CAD build for the part. Positions are in the model's coordinates, mm. Face numbers are marked on the shaded views. A direction names the side the tool comes from. Coordinates: 2 decimals unless noted, no trailing zeros. Order: outer loops, then holes, each group sorted by start corner. A loop starts at its lowest first (then second) coordinate and runs counter-clockwise, first axis right, second up. Notation, with made-up numbers: M 79,11.5 L 134,11.5 A20 ccw 134,44.5 Z; hole C 49,80 d8. An arc over 180 degrees is marked long. Write item = value, one per line.
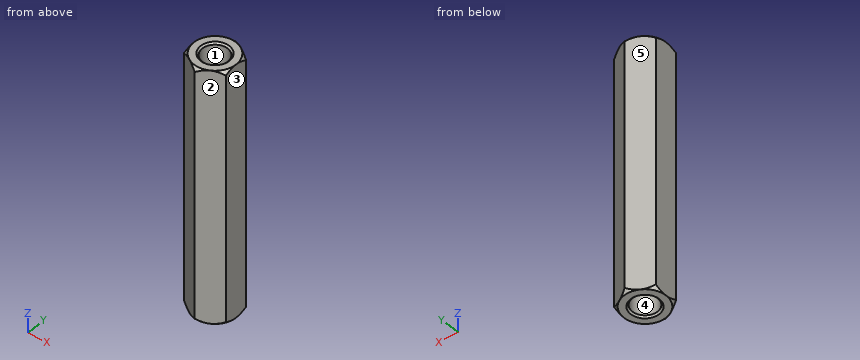
Autodesk Inventor part; units mm, degrees
ref_plane "Pracovní rovina1" through (0, 0, 15) normal (0, 0, -1) x (-1, 0, 0)
ref_plane "YZ Plane" through (0, 0, 0) normal (1, 0, 0) x (0, 1, 0)
ref_plane "XZ Plane" through (0, 0, 0) normal (0, 1, 0) x (-1, 0, 0)
sketch "Náčrt1" plane through (0, 0, 0) normal (0, 0, 1) x (1, 0, 0)
  line L0 (2.5, -1.4434) -> (0, -2.8868)
  line L1 (0, -2.8868) -> (-2.5, -1.4434)
  line L2 (-2.5, -1.4434) -> (-2.5, 1.4434)
  line L3 (-2.5, 1.4434) -> (0, 2.8868)
  line L4 (0, 2.8868) -> (2.5, 1.4434)
  line L5 (2.5, 1.4434) -> (2.5, -1.4434)
  circle A0 centre (0, 0) radius 1.5
  point P0 (2.5, 0)
  dimension "d1" = 3
  dimension "d16" = 5
extrude "Vysunutí1" add sketch "Náčrt1" along normal blind 30
thread "Závit1"
sketch "Náčrt2" plane through (0, 0, 30) normal (0, 0, 1) x (1, 0, 0)
  circle A0 centre (0, 0) radius 2.5
  dimension "d18" = 5
extrude "Vysunutí2" cut sketch "Náčrt2" against normal through all draft 45 keep common part
sketch "Náčrt3" plane through (0, 0, 0) normal (0, 0, -1) x (-1, 0, 0)
  circle A0 centre (0, 0) radius 2.5
  dimension "d17" = 5
extrude "Vysunutí3" cut sketch "Náčrt3" against normal through all draft 45 keep common part
chamfer "Zkosení1" distance 0.2 angle 45 1 edges at (-1.5, 0, 30)
chamfer "Zkosení2" distance 0.2 angle 45 1 edges at (-1.5, 0, 0)
ref_plane "Pracovní rovina1" through (0, 0, 15) normal (0, 0, -1) x (-1, 0, 0)
sketch "Náčrt4" plane through (-2.5, 1.4434, 29.6132) normal (-0.5, 0.8660254, 0) x (0.8660254, 0.5, 0)
  point P0 (1.4434, 29.6132)
sketch "Náčrt5" plane through (0, 0, 15) normal (0, 0, -1) x (-1, 0, 0)
  circle A0 centre (0, 0) radius 1.5
extrude "Vysunutí4" add sketch "Náčrt5" along normal mid plane 8
properties part number "PillarBolt-M3x30" material "Ocel, vysokopevnostní, nízkolegovaná"
(1) Pull direction Y, two halves, no side cores. Call the marked faces 3, 4 and 5: +Y half, -Y half, draft (parallel to the pull), parting line (faces both ways), or undercut.
Evaluation:
face_3 = draft
face_4 = undercut
face_5 = +Y half
(2) Slice it at A-A, the plane z = 3. Write the cut outline in (x, y), then the cut area to 3 significant figures.
Evaluation:
outline = M -2.5,-1.44 L 0,-2.89 L 2.5,-1.44 L 2.5,1.44 L 0,2.89 L -2.5,1.44 Z; hole C 0,0 d3
area = 14.6 mm²
(3) Wall check: line 1 (X direction, y = 0, z = 23.25); line 2 (Y direction, x = -1, z = 1.5); line 3 (Z direction, x = -1.4, y = 0.25). Give the ranges that are in metal, low to high. Write a range as from..to.
Evaluation:
line_1 = -2.5..-1.5, 1.5..2.5
line_2 = -2.31..-1.12, 1.12..2.31
line_3 = 11..19
(4) Tool access for the marked faces 1 and 2: list every direction of +Z, -Z, +X, -X, +Y, -Y with a clear straight run to the whole face (end or side of a thin tool).
Evaluation:
face_1 = +Z
face_2 = +Z, -Z, +X, -Y
(5) Pin check, flat tip, straight feed: pin 1 Ø0.9 at (x, y) = (0.5, 0.5) entering from +Z. Stop position of the tip, or through.
Evaluation:
pin_1 = 19
